from build123d import *

# Parameters (mm, degrees)
F0_W     = 4
F0_H     = 3.5
F0_W_2   = 11
F0_H_2   = 4
F0_W_3   = 10
F1_DEPTH = 15
F2_DEPTH = 5
F3_R     = 5
F4_R     = 5
F5_SIZE  = 3.5
F7_DEPTH = 40


with BuildPart() as f1:
    # F0 (on Front) → F1 (new body)
    with BuildSketch(Plane.XZ):
        with Locations((-18, -5.75)):
            Rectangle(F0_W, F0_H)
        Polygon((16, -4), (5, -4), (-5, -4), (-5, -7.5), (16, -7.5), align=None)
        Polygon((-16, 4), (-5, 4), (-5, 7.5), (-20, 7.5), (-20, 4), align=None)
        with Locations((-10.5, -5.75)):
            Rectangle(F0_W_2, F0_H)
        Polygon((-16, 0), (-16, 4), (-20, 4), (-20, -4), (-16, -4), align=None)
        Polygon((-5, 4), (5, 4), (16, 4), (20, 4), (20, 7.5), (-5, 7.5), align=None)
        with Locations((-10.5, 2)):
            Rectangle(F0_W_2, F0_H_2)
        with Locations((0, 2)):
            Rectangle(F0_W_3, F0_H_2)
        with Locations((-10.5, -2)):
            Rectangle(F0_W_2, F0_H_2)
        with Locations((0, -2)):
            Rectangle(F0_W_3, F0_H_2)
    extrude(amount=F1_DEPTH)

    # F0 (on Front) → F2 (join)
    with BuildSketch(Plane.XZ):
        with Locations((-10.5, 2)):
            Rectangle(F0_W_2, F0_H_2)
        with Locations((0, 2)):
            Rectangle(F0_W_3, F0_H_2)
        with Locations((0, -2)):
            Rectangle(F0_W_3, F0_H_2)
        with Locations((10.5, 2)):
            Rectangle(F0_W_2, F0_H_2)
        with Locations((-10.5, -2)):
            Rectangle(F0_W_2, F0_H_2)
        with Locations((10.5, -2)):
            Rectangle(F0_W_2, F0_H_2)
        Polygon((-5, 4), (5, 4), (16, 4), (20, 4), (20, 7.5), (-5, 7.5), align=None)
        Polygon((16, -4), (5, -4), (-5, -4), (-5, -7.5), (16, -7.5), align=None)
        with Locations((-10.5, -5.75)):
            Rectangle(F0_W_2, F0_H)
        with Locations((-18, -5.75)):
            Rectangle(F0_W, F0_H)
        Polygon((-16, 0), (-16, 4), (-20, 4), (-20, -4), (-16, -4), align=None)
        Polygon((-16, 4), (-5, 4), (-5, 7.5), (-20, 7.5), (-20, 4), align=None)
    extrude(amount=F2_DEPTH)

    # F3
    f3_edges = [f1.edges().sort_by_distance(p)[0] for p in [
        (-20, -7.5, 7.5),
    ]]
    fillet(f3_edges, radius=F3_R)

    # F4
    f4_edges = [f1.edges().sort_by_distance(p)[0] for p in [
        (-20, -7.5, -7.5),
    ]]
    fillet(f4_edges, radius=F4_R)

    # F5
    f5_edges = [f1.edges().sort_by_distance(p)[0] for p in [
        (16, -7.5, -7.5),
    ]]
    chamfer(f5_edges, length=F5_SIZE)

    # F6 (on face) → F7 (cut)
    with BuildSketch(Plane.YZ.offset(20)):
        with BuildLine():
            ThreePointArc((-6.5, -5.75), (-6.7928932188, -5.0428932188), (-7.5, -4.75))
            Line((-7.5, -4.75), (-7.5, -6.75))
            ThreePointArc((-7.5, -6.75), (-6.7928932188, -6.4571067812), (-6.5, -5.75))
        make_face()
        with BuildLine():
            Line((-7.5, -6.75), (-7.5, -4.75))
            ThreePointArc((-7.5, -4.75), (-8.5, -5.75), (-7.5, -6.75))
        make_face()
        with BuildLine():
            ThreePointArc((-7.5, 6.75), (-8.5, 5.75), (-7.5, 4.75))
            Line((-7.5, 4.75), (-7.5, 6.75))
        make_face()
        with BuildLine():
            Line((-7.5, 6.75), (-7.5, 4.75))
            ThreePointArc((-7.5, 4.75), (-6.7928932188, 5.0428932188), (-6.5, 5.75))
            ThreePointArc((-6.5, 5.75), (-6.7928932188, 6.4571067812), (-7.5, 6.75))
        make_face()
    extrude(amount=-F7_DEPTH, mode=Mode.SUBTRACT)


solid = f1.part
Could you check a few things on this model? Use its own coordinates, in mm. A direction names the side the tool comes from. Coordinates: 2 decimals unless noted, no trailing zeros. Write each loop counter-clockwise with the first axis right and the second up, starting at its lowest first coordinate (ties: lowest second). Pieces come first, ordered by that corner, then holes. Notation, with made-up numbers: (35.25, -26) - (54.25, -26) arc R12 cw to (54.25, -4) - close; hole circle Ø5 at (25, 28). An arc over 180 degrees is marked (long way). Put each result on its own line as item: value. Start each with the question number.
Q1. I'm going to push flat-ended pins straight in: P1, Ø2, axis at y = -2, z = -5, coming from the -X side; P2, Ø4, axis at y = -3.5, z = -2, coming from the +X side; P3, Ø2.5, axis at y = -9, z = -1, coming from the +X side. Where does each tip first touch, or does it pass through?
Q2. Thinking about a two-plate mould opening in Z: for faces 1 (the flat face through (10, -5, 0)), 2 (the flat face through (-1, -7, -7.5)), 3 (the flat face through (20, -7.4, 4.6)), which applies, pulls with the +Z half, pulls with the -Z half, needs draft (parallel to the pull), parting line crosses it, or undercut?
Q3. I want a section at B-B on y = -2.5. Write out the boundary of the cut face in (x, z).
Q4. I want a section at D-D on x = -10. Write out the boundary of the cut face in (y, z).
Q5. I want a section at C-C on z = 1. Write out the boundary of the cut face in (x, y), plus the area to 3 significant figures.
Q6. Please list where these lines run through material, in increasing order: L1, parallel to Z at x = -6, y = -7.5; L2, parallel to Y at x = 5.5, z = 5.75; L3, parallel to Z at x = 9, y = -13.75.
Q7. Which directions (+Z, -Z, +X, -X, +Y, -Y) give clear straight access to the entire face, cutting with the end or side of a thin tool? Please do faces 4 (the flat face through (5, -10, 0)), 5 (the flat face through (16, -2, 0)), 6 (the flat face through (3, -7, 7.5)).
Q8. I want a section at A-A on x = 9. Write out the boundary of the cut face in (y, z), plus the area to 3 significant figures.
Checks:
1. P1: x = -19.77
1. P2: x = 16
1. P3: x = 5
2. face 1: undercut
2. face 2: pulls with the -Z half
2. face 3: needs draft
3. outline: (-20, -2.5) arc R5 ccw to (-15, -7.5) - (12.5, -7.5) - (16, -4) - (16, 4) - (20, 4) - (20, 7.5) - (-15, 7.5) arc R5 ccw to (-20, 2.5) - close
4. outline: (-15, -7.5) - (0, -7.5) - (0, 7.5) - (-15, 7.5) - close; hole circle Ø2 at (-7.5, -5.75); hole circle Ø2 at (-7.5, 5.75)
5. outline: (-20, -15) - (5, -15) - (5, -5) - (16, -5) - (16, 0) - (-20, 0) - close
5. area: 430 mm²
6. L1: -7.5 to -6.75, -4.75 to 4.75, 6.75 to 7.5
6. L2: -15 to -8.5, -6.5 to 0
6. L3: -7.5 to -4, 4 to 7.5
7. face 4: +X, -Y
7. face 5: -Z, +X, +Y, -Y
7. face 6: +Z, +X, -X, +Y, -Y
8. outline: (-15, -7.5) - (0, -7.5) - (0, 7.5) - (-15, 7.5) - (-15, 4) - (-5, 4) - (-5, -4) - (-15, -4) - close; hole circle Ø2 at (-7.5, -5.75); hole circle Ø2 at (-7.5, 5.75)
8. area: 139 mm²
